```python
from build123d import *

# Parameters (mm, degrees)
F0_W         = 34.9
F0_H         = 44.5
F1_DEPTH     = 57
F2_W         = 30.5
F2_H         = 40.8
F3_DEPTH     = 55
F5_DEPTH     = 57.001
F6_W         = 1.75
F6_H         = 38.5
F7_DEPTH     = 34.901
F8_W         = 15.9
F8_H         = 6.8
F8_W_2       = 32.4
F8_H_2       = 4.6
F9_DEPTH     = 34.901
F10_W        = 34
F10_H        = 4
F11_DEPTH    = 9.3
F12_W        = 34
F12_H        = 4
F13_DEPTH    = 9.3
F14_SIZE     = 9.29999
F15_SIZE     = 1
F16_R        = 2.35
F17_DEPTH    = 4.001
F18_T1_DEPTH = 26.953787589
F18_T3_DEPTH = 26.953787589


# Not quite as in the source:
# - a fillet or chamfer that OpenCascade refuses, or shapes differently, is made with other operations: its cross-section is extruded or revolved along the edge and cut away or added
# - a fillet or chamfer is up to 0.001 mm smaller than in the source, because OpenCascade refuses the exact size


with BuildPart() as f1:
    # F0 (on Top) → F1 (new body)
    with BuildSketch(Plane.XY):
        with Locations((17.45, 22.6589083523)):
            Rectangle(F0_W, F0_H)
    extrude(amount=F1_DEPTH)

    # F2 (on face) → F3 (cut)
    with BuildSketch(Plane(origin=(0, 0, 0), x_dir=(1, 0, 0), z_dir=(0, 0, -1))):
        with Locations((17.45, -22.6589083523)):
            Rectangle(F2_W, F2_H)
    extrude(amount=-F3_DEPTH, mode=Mode.SUBTRACT)

    # F4 (on face) → F5 (cut, through all)
    with BuildSketch(Plane.XY.offset(57)):
        with BuildLine():
            Line((18.95, 33.2867875695), (18.95, 33.7075508028))
            ThreePointArc((18.95, 33.7075508028), (17.45, 33.8089083523), (15.95, 33.7075508028))
            Line((15.95, 33.7075508028), (15.95, 33.2867875695))
            Line((15.95, 33.2867875695), (18.95, 33.2867875695))
        make_face()
        with BuildLine():
            ThreePointArc((15.95, 33.7075508028), (10.1152368818, 14.2610663676), (28.6, 22.6589083523))
            ThreePointArc((28.6, 22.6589083523), (25.8478419847, 29.9936714704), (18.95, 33.7075508028))
            Line((18.95, 33.7075508028), (18.95, 33.2867875695))
            Line((18.95, 33.2867875695), (15.95, 33.2867875695))
            Line((15.95, 33.2867875695), (15.95, 33.7075508028))
        make_face()
        with BuildLine():
            ThreePointArc((15.95, 33.7075508028), (17.45, 33.8089083523), (18.95, 33.7075508028))
            Line((18.95, 33.7075508028), (18.95, 34.6477875695))
            Line((18.95, 34.6477875695), (15.95, 34.6477875695))
            Line((15.95, 34.6477875695), (15.95, 33.7075508028))
        make_face()
    extrude(amount=-F5_DEPTH, mode=Mode.SUBTRACT)

    # F6 (on face) → F7 (cut, through all)
    with BuildSketch(Plane(origin=(0, 0, 0), x_dir=(0, -1, 0), z_dir=(-1, 0, 0))):
        with Locations((-44.0339083523, 26.15)):
            Rectangle(F6_W, F6_H)
        with Locations((-1.2839083523, 26.15)):
            Rectangle(F6_W, F6_H)
    extrude(amount=-F7_DEPTH, mode=Mode.SUBTRACT)

    # F8 (on face) → F9 (cut, through all)
    with BuildSketch(Plane(origin=(0, 0, 0), x_dir=(0, -1, 0), z_dir=(-1, 0, 0))):
        Polygon((-10.4089083523, 36.8), (-34.9089083523, 36.8), (-34.9089083523, 21.9), (-30.6089083523, 21.9), (-14.7089083523, 21.9), (-10.4089083523, 21.9), align=None)
        with Locations((-22.6589083523, 18.5)):
            Rectangle(F8_W, F8_H)
        with Locations((-22.6589083523, 2.3)):
            Rectangle(F8_W_2, F8_H_2)
        Polygon((-40.0589083523, 4.6), (-38.8589083523, 4.6), (-6.4589083523, 4.6), (-5.2589083523, 4.6), (-5.2589083523, 5.4), (-40.0589083523, 5.4), align=None)
    extrude(amount=-F9_DEPTH, mode=Mode.SUBTRACT)

    # F10 (on face) → F11 (join)
    with BuildSketch(Plane.XZ.offset(-0.4089083523)):
        with Locations((17.45, 2)):
            Rectangle(F10_W, F10_H)
    extrude(amount=F11_DEPTH)

    # F12 (on face) → F13 (join)
    with BuildSketch(Plane(origin=(0, 44.9089083523, 0), x_dir=(-1, 0, 0), z_dir=(0, 1, 0))):
        with Locations((-17.45, 2)):
            Rectangle(F12_W, F12_H)
    extrude(amount=F13_DEPTH)

    # F14 (size 9.3 in the source; OpenCascade refuses exactly that, so slightly less here)
    f14_edges = [f1.edges().sort_by_distance(p)[0] for p in [
        (34.45, 54.208908, 2),
        (0.45, 54.208908, 2),
        (34.45, -8.891092, 2),
        (0.45, -8.891092, 2),
    ]]
    chamfer(f14_edges, length=F14_SIZE)

    # F15
    f15_edges = [f1.edges().sort_by_distance(p)[0] for p in [
        (1.1, 38.858908, 4.6),
        (1.1, 6.458908, 4.6),
        (33.8, 6.458908, 4.6),
        (33.8, 38.858908, 4.6),
    ]]
    chamfer(f15_edges, length=F15_SIZE)

    # F16 (on face) → F17 (cut, through all)
    with BuildSketch(Plane.XY.offset(4)):
        with Locations((17.45, -4.6910916477)):
            Circle(F16_R)
        with Locations((17.45, 50.0089083523)):
            Circle(F16_R)
    extrude(amount=-F17_DEPTH, mode=Mode.SUBTRACT)

    # F18: fillet of radius 5 on 4 edges, made by hand

    # F18_s2 → F18_t1 (cut)
    with BuildSketch(Plane.YZ.offset(-12.3768937945)):
        with BuildLine():
            ThreePointArc((30.6089083523, 16.9492424822), (31.8339911346, 20.2279617444), (34.9089083523, 21.9))
            Line((34.9089083523, 21.9), (30.6089083523, 21.9))
            Line((30.6089083523, 21.9), (30.6089083523, 16.9492424822))
        make_face()
        with BuildLine():
            ThreePointArc((10.4089083523, 21.9), (13.4838255699, 20.2279617444), (14.7089083523, 16.9492424822))
            Line((14.7089083523, 16.9492424822), (14.7089083523, 21.9))
            Line((14.7089083523, 21.9), (10.4089083523, 21.9))
        make_face()
    extrude(amount=F18_T1_DEPTH, mode=Mode.SUBTRACT)

    # F18_s4 → F18_t3 (cut)
    with BuildSketch(Plane.YZ.offset(20.3231062055)):
        with BuildLine():
            ThreePointArc((14.7089083523, 16.9492424822), (13.4838255699, 20.2279617444), (10.4089083523, 21.9))
            Line((10.4089083523, 21.9), (14.7089083523, 21.9))
            Line((14.7089083523, 21.9), (14.7089083523, 16.9492424822))
        make_face()
        with BuildLine():
            ThreePointArc((34.9089083523, 21.9), (31.8339911346, 20.2279617444), (30.6089083523, 16.9492424822))
            Line((30.6089083523, 16.9492424822), (30.6089083523, 21.9))
            Line((30.6089083523, 21.9), (34.9089083523, 21.9))
        make_face()
    extrude(amount=F18_T3_DEPTH, mode=Mode.SUBTRACT)


solid = f1.part
```
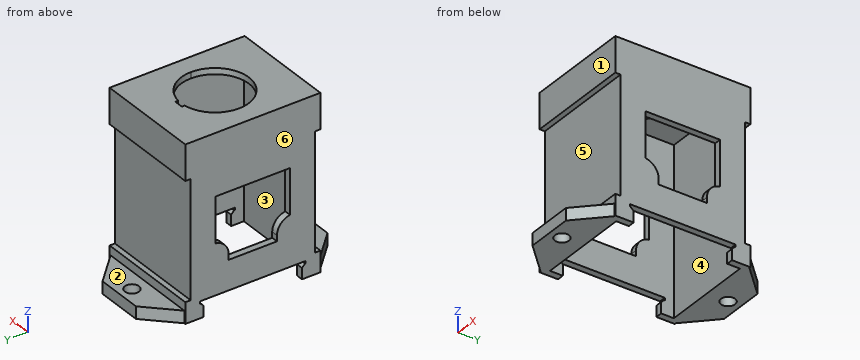
Geometry check sheet. Reference: the model listing, model coordinates, mm. Face numbers are marked on the shaded views. A direction names the side the tool comes from. Coordinates: 2 decimals unless noted, no trailing zeros. Order: outer loops, then holes, each group sorted by start corner. A loop starts at its lowest first (then second) coordinate and runs counter-clockwise, first axis right, second up. Notation, with made-up numbers: M 33.5,84 L 80.5,84 A5 cw 80.5,90 Z; hole C 17.25,-34 d5. An arc over 180 degrees is marked long. Answer as a JSON object with one key per item and string values.
Q1. Cross-section at A-A on z = 44. Record the cut outline in (x, y), and give its area (4 significant figures).
Results are:
{"outline": "M 0,2.16 L 34.9,2.16 L 34.9,43.16 L 0,43.16 Z; hole M 2.2,2.26 L 32.7,2.26 L 32.7,43.06 L 2.2,43.06 Z", "area": "186.5 mm²"}
Q2. Depth check by flat-ended pin: pin 1 Ø10 at (y, z) = (8.5, 35) entering from -X; pin 2 Ø1 at (x, z) = (15, 22.5) entering from -Y; pin 3 Ø2.5 at (x, z) = (1.5, 2) entering from +Y; pin 4 Ø2 at (x, z) = (1, 16) entering from +Y. Enter the tip coordinate at first touch or a pass-through.
Results are:
{"pin 1": "stops at x = 0", "pin 2": "stops at y = 2.16", "pin 3": "stops at y = 47.21", "pin 4": "stops at y = 43.16"}
Q3. Release check for a two-part mould opening along X. For the marked faces 4, 5 and 6 record: released by +X, released by -X, zero draft, split by the parting line, or undercut.
Results are:
{"face 4": "undercut", "face 5": "zero draft", "face 6": "released by -X"}
Q4. Cross-section at B-B on x = 17.45. Give the number of separate pieces and of enclosed holes in the cut face, and give its area (3 significant figures).
Results are:
{"separate pieces": "4", "enclosed holes": "0", "area": "148 mm²"}
Q5. Cross-section at D-D on z = 18. Record the cut outline in (x, y), and give its area (3 significant figures).
Results are:
{"outline": "M 0,2.16 L 34.9,2.16 L 34.9,14.6 L 32.7,14.6 L 32.7,2.26 L 2.2,2.26 L 2.2,14.6 L 0,14.6 Z; M 0,30.72 L 2.2,30.72 L 2.2,43.06 L 32.7,43.06 L 32.7,30.72 L 34.9,30.72 L 34.9,43.16 L 0,43.16 Z", "area": "116 mm²"}
Q6. Cross-section at C-C on x = 13.5. Record the cut outline in (y, z), and give its area (3 significant figures).
Results are:
{"outline": "M -8.89,0 L 2.26,0 L 2.26,55 L 12.23,55 L 12.23,57 L 0.41,57 L 0.41,45.4 L 2.16,45.4 L 2.16,6.9 L 0.41,6.9 L 0.41,4 L -8.89,4 Z; M 33.09,55 L 43.06,55 L 43.06,0 L 54.21,0 L 54.21,4 L 44.91,4 L 44.91,6.9 L 43.16,6.9 L 43.16,45.4 L 44.91,45.4 L 44.91,57 L 33.09,57 Z", "area": "190 mm²"}
Q7. Tool access check on the marked faces 1, 2 and 3. Record the directions out of +Z, -Z, +X, -X, +Y, -Y that give a thin tool (end or side, any length) a straight path to the whole face; none if there is none.
Results are:
{"face 1": "+Z, +X, -X, -Y", "face 2": "+Z, +X, -X, +Y", "face 3": "-Z"}
Q8. Scan lines: line 1 (X direction, y = 3.5, z = 47.5); line 2 (Y direction, x = 18.5, z = 49); line 3 (Y direction, x = 17.45, z = 2.25). Record each from-to range of solid material in increasing order.
Results are:
{"line 1": "x = 0 to 2.2, 32.7 to 34.9", "line 2": "y = 0.41 to 2.26, 43.06 to 44.91", "line 3": "y = -8.89 to -7.04, -2.34 to 2.26, 43.06 to 47.66, 52.36 to 54.21"}
